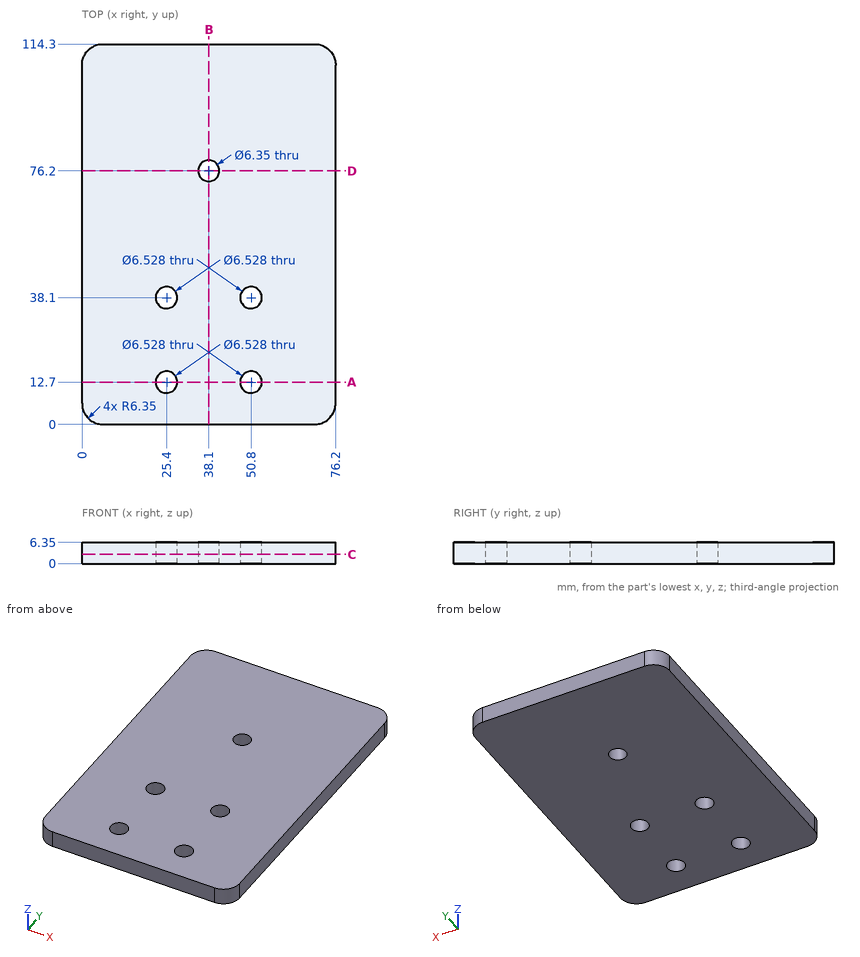
Design review of the part shown in the three views and the two pictorial views. Dimensions are in mm from the part's minimum x, y and z. Round coordinates to 2 decimals unless told otherwise and drop trailing zeros. Loops run counter-clockwise (first coordinate to the right, second up) from the corner with the lowest first, then second, coordinate; pieces in that order, holes last.
Q1. Add section D-D on y = 76.2. Write out the cut boundary in (x, z) (3 decimals).
Result sheet:
outline: (0, 0) - (34.925, 0) - (34.925, 6.35) - (0, 6.35) - close; (41.275, 0) - (76.2, 0) - (76.2, 6.35) - (41.275, 6.35) - close
Q2. Add section C-C on z = 2.75. Give the number of separate pieces and of enclosed holes in the cut face, plus the area to 3 significant figures.
Result sheet:
separate pieces: 1
enclosed holes: 5
area: 8,510 mm2
Q3. To check wall thickness, follow line 1 along Y through (x, z) = (25.4, 3.5); line 2 along Y through (x, z) = (38.1, 3.5) (3 decimals); line 3 along X through (y, z) = (10.5, 0.5). State the ranges of each line that lie inside material, in increasing order.
Result sheet:
line 1: y = 0 to 9.44, 15.96 to 34.84, 41.36 to 114.3
line 2: y = 0 to 73.025, 79.375 to 114.3
line 3: x = 0 to 22.99, 27.81 to 48.39, 53.21 to 76.2
Q4. Add section B-B on x = 38.1. Write out the cut boundary in (y, z) (3 decimals).
Result sheet:
outline: (0, 0) - (73.025, 0) - (73.025, 6.35) - (0, 6.35) - close; (79.375, 0) - (114.3, 0) - (114.3, 6.35) - (79.375, 6.35) - close
Q5. Add section A-A on y = 12.7. Write out the cut boundary in (x, z).
Result sheet:
outline: (0, 0) - (22.14, 0) - (22.14, 6.35) - (0, 6.35) - close; (28.66, 0) - (47.54, 0) - (47.54, 6.35) - (28.66, 6.35) - close; (54.06, 0) - (76.2, 0) - (76.2, 6.35) - (54.06, 6.35) - close
